from build123d import *

# Parameters (mm, degrees)
SKETCH1_R           = 0.75
BOSS_EXTRUDE2_DEPTH = 0.3


with BuildPart() as part:
    # Sketch1 → Boss-Extrude2 (new body)
    with BuildSketch(Plane.XY):
        with BuildLine():
            Line((-0.334323817, 1.971858916), (-0.602966855, 6.919879094))
            ThreePointArc((-0.602966855, 6.919879094), (-0.608561245, 7.18473737), (-0.596611597, 7.449385078))
            Line((-0.596611597, 7.449385078), (-0.156118862, 13.067687454))
            ThreePointArc((-0.156118862, 13.067687454), (-0.151530301, 13.145790905), (-0.15, 13.224014062))
            Line((-0.15, 13.224014062), (-0.15, 19.026340954))
            ThreePointArc((-0.15, 19.026340954), (-1.930835311, 21.281447203), (-0.868120306, 23.951187906))
            ThreePointArc((-0.868120306, 23.951187906), (-0.691943741, 24.15713708), (-0.607202, 24.414570725))
            Line((-0.607202, 24.414570725), (-0.100615971, 28.506000973))
            Line((-0.100615971, 28.506000973), (0.607202, 24.414570725))
            ThreePointArc((0.607202, 24.414570725), (0.691943741, 24.15713708), (0.868120306, 23.951187906))
            ThreePointArc((0.868120306, 23.951187906), (1.930835311, 21.281447203), (0.15, 19.026340954))
            Line((0.15, 19.026340954), (0.15, 13.224014062))
            ThreePointArc((0.15, 13.224014062), (0.151530301, 13.145790905), (0.156118862, 13.067687454))
            Line((0.156118862, 13.067687454), (0.596611597, 7.449385078))
            ThreePointArc((0.596611597, 7.449385078), (0.608561245, 7.18473737), (0.602966855, 6.919879094))
            Line((0.602966855, 6.919879094), (0.334323817, 1.971858916))
            ThreePointArc((0.334323817, 1.971858916), (0, -2), (-0.334323817, 1.971858916))
        make_face()
        Circle(SKETCH1_R, mode=Mode.SUBTRACT)
    extrude(amount=BOSS_EXTRUDE2_DEPTH)


solid = part.part
Here's how the part is built. I have some questions about the finished solid (model axes, mm). Coordinates: 2 decimals unless noted, no trailing zeros. Order: outer loops, then holes, each group sorted by start corner. A loop starts at its lowest first (then second) coordinate and runs counter-clockwise, first axis right, second up. Notation, with made-up numbers: (72.5, -37.5) - (101.5, -37.5) arc R23 cw to (101.5, 0.5) - close; hole circle Ø6 at (50, 86). An arc over 180 degrees is marked (long way). Use CSV: the item, a comma, the result in double quotes. Start each with the question number.
1. I'm going to push a flat-ended pin straight in: pin 1 (2 mm diameter, centred on x = 0.5, y = 2.5, fed in from -Z). Where does the tip first touch, or does it pass through?
2. Please list where these lines run through material, in increasing order: line 1 (X direction, y = -0.5, z = 0.25); line 2 (X direction, y = 14.5, z = 0.2); line 3 (Y direction, x = -1.2, z = 0.15). Write a range as from..to.
3. Suppose I cut it at B-B on z = 0.1. List the corners of the cut face in (x, y) for me, then the cut area to 3 significant figures.
4. Suppose I cut it at A-A on y = 0. List the corners of the cut face in (x, z) for me, then the cut area to 3 significant figures.
Output:
1,pin 1,"stops at z = 0"
2,line 1,"x = -1.94..-0.56, 0.56..1.94"
2,line 2,"x = -0.15..0.15"
2,line 3,"y = -1.6..1.6, 19.75..23.64"
3,outline,"(-0.87, 23.95) arc R2.87 ccw to (-0.15, 19.03) - (-0.15, 13.22) arc R2 cw to (-0.16, 13.07) - (-0.6, 7.45) arc R4 ccw to (-0.6, 6.92) - (-0.33, 1.97) arc R2 ccw (long way) to (0.33, 1.97) - (0.6, 6.92) arc R4 ccw to (0.6, 7.45) - (0.16, 13.07) arc R2 cw to (0.15, 13.22) - (0.15, 19.03) arc R2.87 ccw to (0.87, 23.95) arc R0.7 cw to (0.61, 24.41) - (-0.1, 28.51) - (-0.61, 24.41) arc R0.7 cw to start; hole circle Ø1.5 at (0, 0)"
3,area,"40.4 mm2"
4,outline,"(-2, 0) - (-0.75, 0) - (-0.75, 0.3) - (-2, 0.3) - close; (0.75, 0) - (2, 0) - (2, 0.3) - (0.75, 0.3) - close"
4,area,"0.750 mm2"
